```python
from build123d import *

# Parameters (mm, degrees)
BOSS_EXTRUDE1_DEPTH = 42
BOSS_EXTRUDE2_DEPTH = 4.75
CUT_EXTRUDE1_DEPTH  = 9.5
CUT_EXTRUDE2_DEPTH  = 9.5
FILLET6_R           = 2
FILLET7_START       = -1
FILLET7_DEPTH       = 44
FILLET8_START       = -1
FILLET8_DEPTH       = 44
CHAMFER1_SIZE       = 2
CHAMFER2_SIZE       = 3
CHAMFER3_SIZE       = 2


with BuildPart() as part:
    # Sketch1 → Boss-Extrude1 (new body)
    with BuildSketch(Plane.XY):
        Polygon((0, 0), (-41.3, 0), (-41.3, 9.5), (-9.5, 9.5), (-9.5, 41.3), (0, 41.3), align=None)
    extrude(amount=BOSS_EXTRUDE1_DEPTH)

    # Sketch2 → Boss-Extrude2 (add)
    with BuildSketch(Plane.XY.offset(42)):
        Polygon((-41.3, 9.5), (-9.5, 41.3), (-9.5, 9.5), align=None)
    boss_extrude2 = extrude(amount=-BOSS_EXTRUDE2_DEPTH)

    # Mirror1: Boss-Extrude2 across plane
    add(boss_extrude2.mirror(Plane.XY.offset(21)))

    # Sketch3 → Cut-Extrude1 (cut)
    with BuildSketch(Plane.ZY.offset(9.5)):
        with BuildLine():
            Line((17, 16.15), (25, 16.15))
            ThreePointArc((25, 16.15), (25.707106781, 16.442893219), (26, 17.15))
            Line((26, 17.15), (26, 33.65))
            ThreePointArc((26, 33.65), (25.707106781, 34.357106781), (25, 34.65))
            Line((25, 34.65), (17, 34.65))
            ThreePointArc((17, 34.65), (16.292893219, 34.357106781), (16, 33.65))
            Line((16, 33.65), (16, 17.15))
            ThreePointArc((16, 17.15), (16.292893219, 16.442893219), (17, 16.15))
        make_face()
    extrude(amount=-CUT_EXTRUDE1_DEPTH, mode=Mode.SUBTRACT)

    # Sketch4 → Cut-Extrude2 (cut)
    with BuildSketch(Plane(origin=(0, 9.5, 0), x_dir=(1, 0, 0), z_dir=(0, 1, 0))):
        with BuildLine():
            Line((-33.65, -26), (-17.15, -26))
            ThreePointArc((-17.15, -26), (-16.442893219, -25.707106781), (-16.15, -25))
            Line((-16.15, -25), (-16.15, -17))
            ThreePointArc((-16.15, -17), (-16.442893219, -16.292893219), (-17.15, -16))
            Line((-17.15, -16), (-33.65, -16))
            ThreePointArc((-33.65, -16), (-34.357106781, -16.292893219), (-34.65, -17))
            Line((-34.65, -17), (-34.65, -25))
            ThreePointArc((-34.65, -25), (-34.357106781, -25.707106781), (-33.65, -26))
        make_face()
    extrude(amount=-CUT_EXTRUDE2_DEPTH, mode=Mode.SUBTRACT)

    # Fillet6
    fillet6_edges = [part.edges().sort_by_distance(p)[0] for p in [
        (-9.5, 9.5, 21),
    ]]
    fillet(fillet6_edges, radius=FILLET6_R)

    # Fillet7: read off the stored shape, not the designer's step
    # Fillet7 outline → Fillet7 (cut)
    with BuildSketch(Plane.XY.offset(FILLET7_START)):
        with BuildLine():
            Line((-9.5, 41.3), (-10.378679656, 40.421320344))
            ThreePointArc((-10.378679656, 40.421320344), (-9.40540961, 41.071638598), (-8.257359313, 41.3))
            Line((-8.257359313, 41.3), (-9.5, 41.3))
        make_face()
    extrude(amount=FILLET7_DEPTH, mode=Mode.SUBTRACT)

    # Fillet8: read off the stored shape, not the designer's step
    # Fillet8 outline → Fillet8 (cut)
    with BuildSketch(Plane.XY.offset(FILLET8_START)):
        with BuildLine():
            Line((-40.421320344, 10.378679656), (-41.3, 9.5))
            Line((-41.3, 9.5), (-41.3, 8.257359313))
            ThreePointArc((-41.3, 8.257359313), (-41.071638598, 9.40540961), (-40.421320344, 10.378679656))
        make_face()
    extrude(amount=FILLET8_DEPTH, mode=Mode.SUBTRACT)

    # Chamfer1
    chamfer1_edges = [part.edges().sort_by_distance(p)[0] for p in [
        (0, 41.3, 21),
    ]]
    chamfer(chamfer1_edges, length=CHAMFER1_SIZE)

    # Chamfer2
    chamfer2_edges = [part.edges().sort_by_distance(p)[0] for p in [
        (0, 0, 21),
    ]]
    chamfer(chamfer2_edges, length=CHAMFER2_SIZE)

    # Chamfer3
    chamfer3_edges = [part.edges().sort_by_distance(p)[0] for p in [
        (-41.3, 0, 21),
    ]]
    chamfer(chamfer3_edges, length=CHAMFER3_SIZE)


solid = part.part
```
Geometry: final body of the model. Coordinates: model frame, mm. A direction names the side the tool comes from. Coordinates: 2 decimals unless noted, no trailing zeros. Loops run counter-clockwise (first coordinate to the right, second up) from the corner with the lowest first, then second, coordinate; pieces in that order, holes last. Notation, with made-up numbers: (79.25, 41.5) -> (97.25, 41.5) arc R30 cw to (97.25, 76.5) -> close; hole circle Ø10 at (16.25, 28.25). An arc over 180 degrees is marked (long way). Use a Markdown table: item, result. Add a question column.
(1) Mould query, pull axis Z, two halves, no side actions, for faces 1 (the flat face through (-5, 25, 26)), 2 (the flat face through (-16, 16, 0)), 3 (the flat face through (-25.6, 25.2, 2.3)). Classes: pulls with the +Z half, pulls with the -Z half, needs draft (parallel to the pull), parting line crosses it, or undercut.
(2) Line query: line 1 along Z through (x, y) = (-14, 27); line 2 along X through (y, z) = (36.5, 25); line 3 along Y through (x, z) = (-15, 24.5). Output: solid intervals per line, ascending.
(3) Section query A-A, the plane y = 24.5. Return loops of the section in (x, z).
(4) Section query D-D, the plane z = 11. Return loops of the section in (x, y).
(5) Section query B-B, the plane x = -23. Return loops of the section in (y, z).
(6) Access query for faces 4 (the flat face through (-5, 16.15, 21)), 5 (the flat face through (-13, 0, 21)), 6 (the flat face through (-34.65, 5, 21)), 7 (the cylindrical face through (-9.175, 41.156, 20.706)), 8 (the flat face through (-22, 22, 4.75)). Directions: +Z, -Z, +X, -X, +Y, -Y. A direction counts if a zero-diameter tool reaches every point of the face in a straight line with its end or side. Return the directions, or none.
(7) Section query C-C, the plane z = 21.5. Return loops of the section in (x, y).
(8) Pin query (flat end, axial travel): pin 1 Ø23.5 at (y, z) = (20.5, 16.5) entering from -X; pin 2 Ø3 at (y, z) = (24.5, 7) entering from -X; pin 3 Ø9 at (x, z) = (-24.5, 18) entering from +Y. Return the tip coordinate at first contact, or that it passes through.
Answer:
| question | item | result |
|---|---|---|
| 1 | face 1 | undercut |
| 1 | face 2 | pulls with the -Z half |
| 1 | face 3 | needs draft |
| 2 | line 1 | z = 0 to 4.75, 37.25 to 42 |
| 2 | line 2 | x = -9.5 to 0 |
| 2 | line 3 | y = 0 to 9.5 |
| 3 | outline | (-26.3, 0) -> (0, 0) -> (0, 16) -> (-9.5, 16) -> (-9.5, 4.75) -> (-26.3, 4.75) -> close; (-26.3, 37.25) -> (-9.5, 37.25) -> (-9.5, 26) -> (0, 26) -> (0, 42) -> (-26.3, 42) -> close |
| 4 | outline | (-41.3, 2) -> (-39.3, 0) -> (-3, 0) -> (0, 3) -> (0, 39.3) -> (-2, 41.3) -> (-8.26, 41.3) arc R3 ccw to (-9.5, 41.03) -> (-9.5, 11.5) arc R2 cw to (-11.5, 9.5) -> (-41.03, 9.5) arc R3 ccw to (-41.3, 8.26) -> close |
| 5 | outline | (0, 0) -> (27.8, 0) -> (27.8, 4.75) -> (9.5, 4.75) -> (9.5, 16) -> (0, 16) -> close; (0, 26) -> (9.5, 26) -> (9.5, 37.25) -> (27.8, 37.25) -> (27.8, 42) -> (0, 42) -> close |
| 6 | face 4 | +X, -X |
| 6 | face 5 | +Z, -Z, +X, -X, -Y |
| 6 | face 6 | +Y, -Y |
| 6 | face 7 | +Z, -Z, -X, +Y |
| 6 | face 8 | -X, +Y |
| 7 | outline | (-41.3, 2) -> (-39.3, 0) -> (-34.65, 0) -> (-34.65, 9.5) -> (-41.03, 9.5) arc R3 ccw to (-41.3, 8.26) -> close; (-16.15, 0) -> (-3, 0) -> (0, 3) -> (0, 16.15) -> (-9.5, 16.15) -> (-9.5, 11.5) arc R2 cw to (-11.5, 9.5) -> (-16.15, 9.5) -> close; (-9.5, 34.65) -> (0, 34.65) -> (0, 39.3) -> (-2, 41.3) -> (-8.26, 41.3) arc R3 ccw to (-9.5, 41.03) -> close |
| 8 | pin 1 | stops at x = -41.26 |
| 8 | pin 2 | stops at x = -9.5 |
| 8 | pin 3 | stops at y = 9.5 |
